The model under review builds one solid part; all positions refer to its coordinate system, in mm. A direction names the side the tool comes from. Round coordinates to 2 decimals unless told otherwise and drop trailing zeros. Write each loop counter-clockwise with the first axis right and the second up, starting at its lowest first coordinate (ties: lowest second). Pieces come first, ordered by that corner, then holes.
Item 1: Machinability: for faces 1 (the face through (-36, 1, -0.5)), 2 (the face through (34, 36, 0)), which of the approach directions +Z, -Z, +X, -X, +Y, -Y give a long, thin tool a straight path to every point of the face, cutting with its end or side? Answer none if there is none.
Item 2: Add section C-C (z = -0.25). State how many separate pieces and enclosed holes the cut face has, plus the area to 3 significant figures.
Item 3: Add section B-B (x = 8). Give the boundary of the cut face in (y, z).
Item 4: Add section A-A (y = 4). Give the boundary of the cut face in (x, z), plus the area to 3 significant figures.
Item 5: To check wall thickness, follow L1, parallel to Y at x = 30.5, z = 0.05; L2, parallel to Y at x = 0, z = -0.25; L3, parallel to X at y = 47.5, z = -0.2. State the ranges of each line that lie inside material, in increasing order.
```python
from build123d import *

# Parameters (mm, degrees)
SKETCH1_W                   = 81
SKETCH1_H                   = 100
BOSS_EXTRUDE1_DEPTH         = 0.5
CUT_EXTRUDE1_DEPTH          = 65.352544627
M1_6_HOLE1_PCBUNION_D       = 1.8
M1_6_HOLE1_PCBUNION_DEPTH   = 100
M1_6_HOLE1_PCBUNION_TIP     = 0.540774557
M1_6_HOLE2_PLATEUNION_D     = 1.8
M1_6_HOLE2_PLATEUNION_DEPTH = 100
M1_6_HOLE2_PLATEUNION_TIP   = 0.540774557
M1_6_HOLE3_TOPUNION_D       = 1.8
M1_6_HOLE3_TOPUNION_DEPTH   = 200
M1_6_HOLE3_TOPUNION_TIP     = 0.540774557
FILLET1_R                   = 0.1


with BuildPart() as part:
    # Sketch1 → Boss-Extrude1 (new, symmetric)
    with BuildSketch(Plane.XY):
        Rectangle(SKETCH1_W, SKETCH1_H)
    extrude(amount=BOSS_EXTRUDE1_DEPTH, both=True)

    # Sketch2 → Cut-Extrude1 (cut, through all)
    with BuildSketch(Plane.XY.offset(0.5)):
        with BuildLine():
            Line((-30, -38), (30, -38))
            ThreePointArc((30, -38), (33.535533906, -36.535533906), (35, -33))
            Line((35, -33), (35, 33))
            ThreePointArc((35, 33), (33.535533906, 36.535533906), (30, 38))
            Line((30, 38), (-30, 38))
            ThreePointArc((-30, 38), (-33.535533906, 36.535533906), (-35, 33))
            Line((-35, 33), (-35, -33))
            ThreePointArc((-35, -33), (-33.535533906, -36.535533906), (-30, -38))
        make_face()
    extrude(amount=-CUT_EXTRUDE1_DEPTH, mode=Mode.SUBTRACT)

    # M1.6 Hole1-PCBUnion
    with Locations(Plane.XY.offset(0.5)):
        with Locations((-30.5, 40.5), (30.5, 40.5), (-30.5, -40.5), (30.5, -40.5)):
            Hole(M1_6_HOLE1_PCBUNION_D / 2, depth=M1_6_HOLE1_PCBUNION_DEPTH)
            with Locations((0, 0, -(M1_6_HOLE1_PCBUNION_DEPTH + M1_6_HOLE1_PCBUNION_TIP / 2))):  # 118° drill point
                Cone(0, M1_6_HOLE1_PCBUNION_D / 2, M1_6_HOLE1_PCBUNION_TIP, mode=Mode.SUBTRACT)

    # M1.6 Hole2-PlateUnion
    with Locations(Plane.XY.offset(0.5)):
        with Locations((-21.5, 47.5), (21.5, 47.5), (-21.5, -47.5), (21.5, -47.5)):
            Hole(M1_6_HOLE2_PLATEUNION_D / 2, depth=M1_6_HOLE2_PLATEUNION_DEPTH)
            with Locations((0, 0, -(M1_6_HOLE2_PLATEUNION_DEPTH + M1_6_HOLE2_PLATEUNION_TIP / 2))):  # 118° drill point
                Cone(0, M1_6_HOLE2_PLATEUNION_D / 2, M1_6_HOLE2_PLATEUNION_TIP, mode=Mode.SUBTRACT)

    # M1.6 Hole3-TopUnion
    with Locations(Plane.XY.offset(0.5)):
        with Locations((0, 47.5), (0, -47.5)):
            Hole(M1_6_HOLE3_TOPUNION_D / 2, depth=M1_6_HOLE3_TOPUNION_DEPTH)
            with Locations((0, 0, -(M1_6_HOLE3_TOPUNION_DEPTH + M1_6_HOLE3_TOPUNION_TIP / 2))):  # 118° drill point
                Cone(0, M1_6_HOLE3_TOPUNION_D / 2, M1_6_HOLE3_TOPUNION_TIP, mode=Mode.SUBTRACT)

    # Fillet1
    fillet1_edges = [part.edges().sort_by_distance(p)[0] for p in [
        (-40.5, 0, 0.5),
        (40.5, 0, 0.5),
        (-40.5, 0, -0.5),
        (40.5, 0, -0.5),
    ]]
    fillet(fillet1_edges, radius=FILLET1_R)


solid = part.part
```
Numbers:
1. face 1: -Z, +X, -X, +Y, -Y
1. face 2: +Z, -Z
2. separate pieces: 1
2. enclosed holes: 11
2. area: 2,780 mm2
3. outline: (-50, -0.5) - (-38, -0.5) - (-38, 0.5) - (-50, 0.5) - close; (38, -0.5) - (50, -0.5) - (50, 0.5) - (38, 0.5) - close
4. outline: (-40.5, -0.4) arc R0.1 ccw to (-40.4, -0.5) - (-35, -0.5) - (-35, 0.5) - (-40.4, 0.5) arc R0.1 ccw to (-40.5, 0.4) - close; (35, -0.5) - (40.4, -0.5) arc R0.1 ccw to (40.5, -0.4) - (40.5, 0.4) arc R0.1 ccw to (40.4, 0.5) - (35, 0.5) - close
4. area: 11.0 mm2
5. L1: y = -50 to -41.4, -39.6 to -37.97, 37.97 to 39.6, 41.4 to 50
5. L2: y = -50 to -48.4, -46.6 to -38, 38 to 46.6, 48.4 to 50
5. L3: x = -40.5 to -22.4, -20.6 to -0.9, 0.9 to 20.6, 22.4 to 40.5
